```python
from build123d import *

# Parameters (mm, degrees)
F0_R      = 25
F2_DEPTH  = 3
F1_R      = 20
F3_DEPTH  = 6
F4_R      = 15
F5_DEPTH  = 9
F6_R      = 10
F7_DEPTH  = 12
F12_R     = 1.5
F13_DEPTH = 30


# Not quite as in the source:
# - a fillet or chamfer that OpenCascade refuses, or shapes differently, is made with other operations: its cross-section is extruded or revolved along the edge and cut away or added


with BuildPart() as f2:
    # F0 (on Top) → F2 (new body)
    with BuildSketch(Plane.XY):
        Circle(F0_R)
    extrude(amount=F2_DEPTH)

    # F1 (on Top) → F3 (join)
    with BuildSketch(Plane.XY):
        Circle(F1_R)
    extrude(amount=F3_DEPTH)

    # F4 (on Top) → F5 (join)
    with BuildSketch(Plane.XY):
        Circle(F4_R)
    extrude(amount=F5_DEPTH)

    # F6 (on Top) → F7 (join)
    with BuildSketch(Plane.XY):
        Circle(F6_R)
    extrude(amount=F7_DEPTH)

    # F8: fillet of radius 5 on 1 edges, made by hand

    # F8_s1 → F8_t2 (revolve, cut)
    with BuildSketch(Plane.XZ):
        with BuildLine():
            ThreePointArc((10, 9), (8.1560370926, 11.1833001327), (5.417424305, 12))
            Line((5.417424305, 12), (10, 12))
            Line((10, 12), (10, 9))
        make_face()
    revolve(axis=Axis((0, 0, 12), (0, 0, 1)), mode=Mode.SUBTRACT)

    # F9: fillet of radius 5 on 1 edges, made by hand

    # F9_s1 → F9_t2 (revolve, cut)
    with BuildSketch(Plane.XZ):
        with BuildLine():
            ThreePointArc((15, 6), (13.1560370926, 8.1833001327), (10.417424305, 9))
            Line((10.417424305, 9), (15, 9))
            Line((15, 9), (15, 6))
        make_face()
    revolve(axis=Axis((0, 0, 9), (0, 0, 1)), mode=Mode.SUBTRACT)

    # F10: fillet of radius 5 on 1 edges, made by hand

    # F10_s1 → F10_t2 (revolve, cut)
    with BuildSketch(Plane.XZ):
        with BuildLine():
            ThreePointArc((20, 3), (18.1560370926, 5.1833001327), (15.417424305, 6))
            Line((15.417424305, 6), (20, 6))
            Line((20, 6), (20, 3))
        make_face()
    revolve(axis=Axis((0, 0, 6), (0, 0, 1)), mode=Mode.SUBTRACT)

    # F11: fillet of radius 5 on 1 edges, made by hand

    # F11_s1 → F11_t2 (revolve, cut)
    with BuildSketch(Plane.XZ):
        with BuildLine():
            ThreePointArc((25, 0), (23.1560370926, 2.1833001327), (20.417424305, 3))
            Line((20.417424305, 3), (25, 3))
            Line((25, 3), (25, 0))
        make_face()
    revolve(axis=Axis((0, 0, 3), (0, 0, 1)), mode=Mode.SUBTRACT)

    # F12 (on Front) → F13 (join)
    with BuildSketch(Plane.XZ):
        with Locations((0, 1.508576342)):
            Circle(F12_R)
    extrude(amount=F13_DEPTH)


solid = f2.part
```
Check sheet for the modelled part. Datum: model origin and axes. Units: mm. A direction names the side the tool comes from. Coordinates: 2 decimals unless noted, no trailing zeros. Order: outer loops, then holes, each group sorted by start corner. A loop starts at its lowest first (then second) coordinate and runs counter-clockwise, first axis right, second up. Notation, with made-up numbers: (-13.5, 18.5) -> (19.5, 18.5) arc R30 ccw to (19.5, 41.5) -> close; hole circle Ø2 at (60.25, -18.75). An arc over 180 degrees is marked (long way). Write item = value, one per line. Start each with the question number.
1) Access from +Z, -Z, +X, -X, +Y, -Y to the whole of each face (thin tool, end or side, straight path). Record for faces 1 (the flat face through (13.5, -15, 3)), 2 (the cylindrical face through (-0.195, -26.039, 2.996)), 3 (the flat face through (0, 0, 12)).
2) Go/stop test with flat-tipped pins: P1, Ø10, axis at x = -18.5, y = 14.5, coming from the +Z side; P2, Ø5, axis at y = 6.5, z = 2.5, coming from the -X side; P3, Ø1.5, axis at y = 6.5, z = 4, coming from the -X side; P4, Ø3, axis at y = 15, z = 9.5, coming from the +X side. Record where each tip stops, or that it passes through.
3) Material ranges on L1, parallel to Z at x = 6, y = 2; L2, parallel to X at y = -11, z = 1.5; L3, parallel to Z at x = -17.5, y = -16, recorded low to high.
4) Cross-section at B-B (z = 10.75). Enter the section's corners in (x, y), then the cut area to 3 significant figures.
5) Cross-section at A-A (z = 8). Enter the section's corners in (x, y).
Ans:
q1.face_1 = +Z
q1.face_2 = -Y
q1.face_3 = +Z, +X, -X, +Y, -Y
q2.P1 = 4.93
q2.P2 = -24.29
q2.P3 = -18.86
q2.P4 = through
q3.L1 = 0 to 11.92
q3.L2 = -21.32 to 21.32
q3.L3 = 0 to 1.76
q4.outline = circle Ø17.45 at (0, 0)
q4.area = 239 mm²
q5.outline = circle Ø26.83 at (0, 0)
